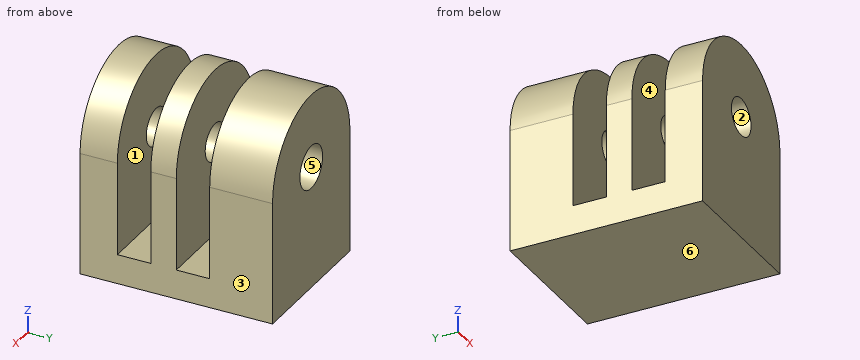
```python
from build123d import *

# Parameters (mm, degrees)
BOX003_W                  = 15
BOX003_H                  = 3.4
BOX003_DEPTH              = 17
ARRAY_Y_COUNT             = 2
ARRAY_Y_PITCH             = 6
CYLINDER002_R             = 2.2
CYLINDER002_DEPTH         = 6
CYLINDER001_R             = 1.9
CYLINDER001_DEPTH         = 15
FUSION001_PLACEMENT_ANGLE = 90
CYLINDER_R                = 7.5
CYLINDER_DEPTH            = 19.6
BOX002_W                  = 15
BOX002_H                  = 19.6
BOX002_DEPTH              = 12.5


with BuildPart() as side_3_extract_cube_array:
    # Box003 → Box003 (new body)
    with BuildSketch(Plane(origin=(-7.5, -7.7, 3), x_dir=(1, 0, 0), z_dir=(0, 0, 1))):
        with Locations((7.5, 1.7)):
            Rectangle(BOX003_W, BOX003_H)
    extrude(amount=BOX003_DEPTH)

    # Array Y: side 3 extract cube array ×2


with BuildPart() as side_3_extract_cube_array_1:
    add(side_3_extract_cube_array.part)
    with Locations(*[(0, i * ARRAY_Y_PITCH, 0) for i in range(1, ARRAY_Y_COUNT)]):
        add(side_3_extract_cube_array.part)


with BuildPart() as side_3_extract_cube_array_2:
    # Array placement: moved
    add(side_3_extract_cube_array_1.part.moved(Location((0, 3, 0))))


with BuildPart() as insert_hole:
    # Cylinder002 → Cylinder002 (new body)
    with BuildSketch(Plane.XY):
        Circle(CYLINDER002_R)
    extrude(amount=CYLINDER002_DEPTH)


with BuildPart() as side_3_extract_fusion:
    # Cylinder001 → Cylinder001 (new body)
    with BuildSketch(Plane.XY.offset(6)):
        Circle(CYLINDER001_R)
    extrude(amount=CYLINDER001_DEPTH)

    # Fusion001: union insert hole
    add(insert_hole.part)


with BuildPart() as side_3_extract_fusion_1:
    # Fusion001 placement: moved
    add(side_3_extract_fusion.part.moved(Location((0, 11.1, 12.5))).rotate(Axis((0, 11.1, 12.5), (1, 0, 0)), FUSION001_PLACEMENT_ANGLE))

    # Fusion002: union side 3 extract cube array
    add(side_3_extract_cube_array_2.part)


with BuildPart() as outer_cylinder:
    # Cylinder → Cylinder (new body)
    with BuildSketch(Plane(origin=(0, 11.1, 12.5), x_dir=(1, 0, 0), z_dir=(0, -1, 0))):
        Circle(CYLINDER_R)
    extrude(amount=CYLINDER_DEPTH)


with BuildPart() as side_3_cut_clone:
    # Box002 → Box002 (new body)
    with BuildSketch(Plane(origin=(-7.5, -8.5, 0), x_dir=(1, 0, 0), z_dir=(0, 0, 1))):
        with Locations((7.5, 9.8)):
            Rectangle(BOX002_W, BOX002_H)
    extrude(amount=BOX002_DEPTH)

    # Fusion: union outer cylinder
    add(outer_cylinder.part)

    # Cut: cut side 3 extract fusion
    add(side_3_extract_fusion_1.part, mode=Mode.SUBTRACT)


solid = side_3_cut_clone.part
```
Input: part model. Units: mm. Frame: model coordinates. Face numbers are marked on the shaded views. A direction names the side the tool comes from. Coordinates: 2 decimals unless noted, no trailing zeros. Loops run counter-clockwise (first coordinate to the right, second up) from the corner with the lowest first, then second, coordinate; pieces in that order, holes last. Notation, with made-up numbers: (18.5, -10) -> (67.5, -10) arc R21 cw to (67.5, 22) -> close; hole circle Ø7 at (-24, 88). An arc over 180 degrees is marked (long way). Use a Markdown table: item, result.
1) Cut plane B-B (x = 0). Return the cut outline in (y, z), then the cut area to 3 significant figures.
Results found:
| item | result |
|---|---|
| outline | (-8.5, 0) -> (11.1, 0) -> (11.1, 10.3) -> (5.1, 10.3) -> (5.1, 10.6) -> (4.7, 10.6) -> (4.7, 3) -> (1.3, 3) -> (1.3, 10.6) -> (-1.3, 10.6) -> (-1.3, 3) -> (-4.7, 3) -> (-4.7, 10.6) -> (-8.5, 10.6) -> close; (-8.5, 14.4) -> (-4.7, 14.4) -> (-4.7, 20) -> (-8.5, 20) -> close; (-1.3, 14.4) -> (1.3, 14.4) -> (1.3, 20) -> (-1.3, 20) -> close; (4.7, 14.4) -> (5.1, 14.4) -> (5.1, 14.7) -> (11.1, 14.7) -> (11.1, 20) -> (4.7, 20) -> close |
| area | 224 mm2 |
2) Pull-direction query (X, two-part tool) for the marked faces 1, 2 and 3; classes: released by +X, released by -X, zero draft, split by the parting line, or undercut.
Results found:
| item | result |
|---|---|
| face 1 | zero draft |
| face 2 | undercut |
| face 3 | released by +X |
3) Cut plane A-A (z = 9.5). Return the cut outline in (x, y).
Results found:
| item | result |
|---|---|
| outline | (-7.5, -8.5) -> (7.5, -8.5) -> (7.5, -4.7) -> (-7.5, -4.7) -> close; (-7.5, -1.3) -> (7.5, -1.3) -> (7.5, 1.3) -> (-7.5, 1.3) -> close; (-7.5, 4.7) -> (7.5, 4.7) -> (7.5, 11.1) -> (-7.5, 11.1) -> close |
4) Contact query for flat-ended pins moving along their axis: pin 1 (6 mm diameter, centred on x = -2, y = 0, fed in from +Z); pin 2 (1.7 mm diameter, centred on x = 2.5, y = 2.5, fed in from +Z). Output: stop coordinate, or through.
Results found:
| item | result |
|---|---|
| pin 1 | stops at z = 20 |
| pin 2 | stops at z = 3 |
5) Access query for the marked faces 4, 5 and 6. Directions: +Z, -Z, +X, -X, +Y, -Y. A direction counts if a zero-diameter tool reaches every point of the face in a straight line with its end or side. Return the directions, or none.
Results found:
| item | result |
|---|---|
| face 4 | +Z, +X, -X |
| face 5 | +Y |
| face 6 | -Z, +X, -X, +Y, -Y |
6) Material intervals for line 1 along Y through (x, z) = (-5, 5); line 2 along X through (y, z) = (0, 12.5); line 3 along Z through (x, y) = (0, 5.05), sorted ascending. Write a range as from..to.
Results found:
| item | result |
|---|---|
| line 1 | y = -8.5..-4.7, -1.3..1.3, 4.7..11.1 |
| line 2 | x = -7.5..-1.9, 1.9..7.5 |
| line 3 | z = 0..10.6, 14.4..20 |
7) Cut plane D-D (x = 6). Return the cut outline in (y, z).
Results found:
| item | result |
|---|---|
| outline | (-8.5, 0) -> (11.1, 0) -> (11.1, 17) -> (4.7, 17) -> (4.7, 3) -> (1.3, 3) -> (1.3, 17) -> (-1.3, 17) -> (-1.3, 3) -> (-4.7, 3) -> (-4.7, 17) -> (-8.5, 17) -> close |
8) Cut plane C-C (y = -6.25). Return the cut outline in (x, z), then the cut area to 3 significant figures.
Results found:
| item | result |
|---|---|
| outline | (-7.5, 0) -> (7.5, 0) -> (7.5, 12.5) arc R7.5 ccw to (-7.5, 12.5) -> close; hole circle Ø3.8 at (0, 12.5) |
| area | 265 mm2 |
